Geometry check sheet. Reference: the model listing, model coordinates, mm. A direction names the side the tool comes from. Coordinates: 2 decimals unless noted, no trailing zeros. Write each loop counter-clockwise with the first axis right and the second up, starting at its lowest first coordinate (ties: lowest second). Pieces come first, ordered by that corner, then holes. Notation, with made-up numbers: (-24.5, 33.5) - (-3.5, 33.5) arc R23 cw to (-3.5, 51.5) - close; hole circle Ø8 at (3, 7.25). An arc over 180 degrees is marked (long way). Answer as a JSON object with one key per item and string values. Group by question number.
from build123d import *
from OCP.BRepFilletAPI import BRepFilletAPI_MakeChamfer

# Parameters (mm, degrees)
BOSS_EXTRUDE1_DEPTH = 2.5
BOSS_EXTRUDE2_DEPTH = 7
SKETCH3_R           = 1.4
CUT_EXTRUDE1_DEPTH  = 2.5
CHAMFER1_SIZE       = 2
CHAMFER1_SIZE2      = 3.464101615


with BuildPart() as part:
    # Sketch1 → Boss-Extrude1 (new body)
    with BuildSketch(Plane(origin=(0, 0, 0), x_dir=(1, 0, 0), z_dir=(0, 1, 0))):
        with BuildLine():
            Line((-7.427428988, -1.040816327), (-4.060327847, -25.068979592))
            ThreePointArc((-4.060327847, -25.068979592), (0, -28.6), (4.060327847, -25.068979592))
            Line((4.060327847, -25.068979592), (7.427428988, -1.040816327))
            ThreePointArc((7.427428988, -1.040816327), (0, 7.5), (-7.427428988, -1.040816327))
        make_face()
    extrude(amount=BOSS_EXTRUDE1_DEPTH)

    # Sketch2 → Boss-Extrude2 (add)
    with BuildSketch(Plane.XZ):
        with BuildLine():
            Line((9.903238651, 1.387755102), (6.53613751, 25.415918367))
            ThreePointArc((6.53613751, 25.415918367), (0, 31.1), (-6.53613751, 25.415918367))
            Line((-6.53613751, 25.415918367), (-9.903238651, 1.387755102))
            ThreePointArc((-9.903238651, 1.387755102), (0, -10), (9.903238651, 1.387755102))
        make_face()
        with BuildLine():
            Line((-7.427428988, 1.040816327), (-4.060327847, 25.068979592))
            ThreePointArc((-4.060327847, 25.068979592), (0, 28.6), (4.060327847, 25.068979592))
            Line((4.060327847, 25.068979592), (7.427428988, 1.040816327))
            ThreePointArc((7.427428988, 1.040816327), (0, -7.5), (-7.427428988, 1.040816327))
        make_face(mode=Mode.SUBTRACT)
    extrude(amount=-BOSS_EXTRUDE2_DEPTH)

    # Sketch3 → Cut-Extrude1 (cut)
    with BuildSketch(Plane(origin=(0, 2.5, 0), x_dir=(1, 0, 0), z_dir=(0, 1, 0))):
        with Locations(Location((0, 0, 0), (0, 0, 270))):
            Circle(SKETCH3_R)
        with Locations(Location((0, -24.5, 0), (0, 0, 270))):
            Circle(SKETCH3_R)
    extrude(amount=-CUT_EXTRUDE1_DEPTH, mode=Mode.SUBTRACT)

    # Chamfer1: one chamfer whose edges measure the first distance from different faces: ONE call of the kernel's chamfer builder (chamfer() names one face for all edges)
    chamfer1_edges_1 = [part.edges().sort_by_distance(p)[0] for p in [
        (0, 0, -10),
    ]]
    chamfer1_side_1 = [part.faces().sort_by_distance(p)[0] for p in [
        (0, 3.5, -10),
    ]]
    chamfer1_edges_2 = [part.edges().sort_by_distance(p)[0] for p in [
        (8.21968808, 0, 13.401836735),
    ]]
    chamfer1_side_2 = [part.faces().sort_by_distance(p)[0] for p in [
        (8.21968808, 3.5, 13.401836735),
    ]]
    chamfer1_edges_3 = [part.edges().sort_by_distance(p)[0] for p in [
        (0, 0, 31.1),
    ]]
    chamfer1_side_3 = [part.faces().sort_by_distance(p)[0] for p in [
        (0, 3.5, 31.1),
    ]]
    chamfer1_edges_4 = [part.edges().sort_by_distance(p)[0] for p in [
        (-8.21968808, 0, 13.401836735),
    ]]
    chamfer1_side_4 = [part.faces().sort_by_distance(p)[0] for p in [
        (-8.21968808, 3.5, 13.401836735),
    ]]
    chamfer1 = BRepFilletAPI_MakeChamfer(part.part.solid().wrapped)
    for e in chamfer1_edges_1:
        chamfer1.Add(CHAMFER1_SIZE, CHAMFER1_SIZE2, e.wrapped, chamfer1_side_1[0].wrapped)  # the first distance lies on this face
    for e in chamfer1_edges_2:
        chamfer1.Add(CHAMFER1_SIZE, CHAMFER1_SIZE2, e.wrapped, chamfer1_side_2[0].wrapped)  # the first distance lies on this face
    for e in chamfer1_edges_3:
        chamfer1.Add(CHAMFER1_SIZE, CHAMFER1_SIZE2, e.wrapped, chamfer1_side_3[0].wrapped)  # the first distance lies on this face
    for e in chamfer1_edges_4:
        chamfer1.Add(CHAMFER1_SIZE, CHAMFER1_SIZE2, e.wrapped, chamfer1_side_4[0].wrapped)  # the first distance lies on this face
    add(Compound.cast(chamfer1.Shape()), mode=Mode.REPLACE)


solid = part.part
(1) Draft check along X on faces 3 (the face through (-0.16, 0.097, -6.702)), 4 (the face through (0, 2.5, 10)), 5 (the face through (8.243, 4.465, 13.234)), 6 (the face through (0.06, 1.27, -1.4)). Enter one of: +X half, -X half, draft (parallel to the pull), parting line (faces both ways), or undercut.
(2) Set-up check for faces 1 (the face through (-0.1, 4.7, 28.6)), 2 (the face through (-0.54, 1.27, 25.79)): record each of +Z, -Z, +X, -X, +Y, -Y from which the full face is reachable in a straight line by a thin tool's end or side.
(3) Section check B-B (y = 4). Record the cut outline in (x, z), and give its area (3 significant figures).
(4) Section check C-C (z = 19). Record the cut outline in (x, y), and give its area (3 significant figures).
(5) Gauge pin test, flat ends, axial feed: pin 1 (1 mm diameter, centred on x = 6.5, y = 2.5, fed in from +Z); pin 2 (1.7 mm diameter, centred on x = 0, z = 24.5, fed in from -Y); pin 3 (2 mm diameter, centred on x = 3, z = 9.5, fed in from +Y); pin 4 (4 mm diameter, centred on y = 2, z = 5, fed in from +X). Record the tip position at first contact, or that the pin passes through.
(6) Section check A-A (z = 0). Record the cut outline in (x, y), and give its area (3 significant figures).
(7) Material ranges on L1, parallel to X at y = 3.7, z = 0; L2, parallel to X at y = 4.25, z = -5; L3, parallel to Y at x = -1, z = -6, recorded low to high. Write a range as [from, to].
(8) Section check D-D (y = 1.25). Record the cut outline in (x, z), and give its area (3 significant figures).
Conclusion:
{
 "1": {"face 3": "parting line", "face 4": "undercut", "face 5": "+X half", "face 6": "undercut"},
 "2": {"face 1": "+Y", "face 2": "+Y, -Y"},
 "3": {"outline": "(-9.9, 1.39) arc R10 ccw (long way) to (9.9, 1.39) - (6.54, 25.42) arc R6.6 ccw to (-6.54, 25.42) - close; hole (-7.43, 1.04) arc R7.5 ccw (long way) to (7.43, 1.04) - (4.06, 25.07) arc R4.1 ccw to (-4.06, 25.07) - close", "area": "234 mm^2"},
 "4": {"outline": "(-7.44, 2) - (-3.94, 0) - (3.94, 0) - (7.44, 2) - (7.44, 7) - (4.91, 7) - (4.91, 2.5) - (-4.91, 2.5) - (-4.91, 7) - (-7.44, 7) - close", "area": "52.9 mm^2"},
 "5": {"pin 1": "stops at z = 27.25", "pin 2": "passes through", "pin 3": "stops at y = 2.5", "pin 4": "stops at x = 9.68"},
 "6": {"outline": "(-10, 2) - (-6.54, 0) - (-1.4, 0) - (-1.4, 2.5) - (-7.5, 2.5) - (-7.5, 7) - (-10, 7) - close; (1.4, 0) - (6.54, 0) - (10, 2) - (10, 7) - (7.5, 7) - (7.5, 2.5) - (1.4, 2.5) - close", "area": "58.6 mm^2"},
 "7": {"L1": "x = [-10, -7.5], [7.5, 10]", "L2": "x = [-8.66, -5.59], [5.59, 8.66]", "L3": "y = [0, 2.5]"},
 "8": {"outline": "(-8.62, 1.21) arc R8.7 ccw (long way) to (8.62, 1.21) - (5.25, 25.24) arc R5.3 ccw to (-5.25, 25.24) - close; hole circle Ø2.8 at (0, 0); hole circle Ø2.8 at (0, 24.5)", "area": "497 mm^2"}
}
